```python
from build123d import *

# Parameters (mm, degrees)
F0_R     = 4
F1_DEPTH = 25


with BuildPart() as f1:
    # F0 (on Front) → F1 (new body)
    with BuildSketch(Plane.XZ):
        with BuildLine():
            ThreePointArc((1.7153142053, -12.3817485509), (9.425800432, -8.2100113408), (12.5, 0))
            ThreePointArc((12.5, 0), (0, 12.5), (-12.5, 0))
            ThreePointArc((-12.5, 0), (-8.8388347648, -8.8388347648), (0, -12.5))
            Line((0, -12.5), (1.7153142053, -12.3817485509))
        make_face()
        Circle(F0_R, mode=Mode.SUBTRACT)
        with BuildLine():
            ThreePointArc((-12.5, 0), (0, 12.5), (12.5, 0))
            ThreePointArc((12.5, 0), (9.425800432, -8.2100113408), (1.7153142053, -12.3817485509))
            Line((1.7153142053, -12.3817485509), (65.5502033349, -7.9810573416))
            ThreePointArc((65.5502033349, -7.9810573416), (57.0047370671, -0.2752646609), (65, 8))
            Line((65, 8), (21.9245263595, 11.0022438251))
            ThreePointArc((21.9245263595, 11.0022438251), (16.3684000055, 13.8215743024), (14.5197193706, 19.771493992))
            Line((14.5197193706, 19.771493992), (18.6307429943, 61.272344506))
            ThreePointArc((18.6307429943, 61.272344506), (0.0177077601, 46.0000082517), (-18.6237623762, 61.2376237624))
            Line((-18.6237623762, 61.2376237624), (-12.5, 0))
        make_face()
        with BuildLine():
            ThreePointArc((0, -12.5), (0.8596927108, -12.4704020963), (1.7153142053, -12.3817485509))
            Line((1.7153142053, -12.3817485509), (0, -12.5))
        make_face()
        with BuildLine():
            Line((-19, 65), (-18.6237623762, 61.2376237624))
            ThreePointArc((-18.6237623762, 61.2376237624), (0.0177077601, 46.0000082517), (18.6307429943, 61.272344506))
            Line((18.6307429943, 61.272344506), (19, 65))
            Line((19, 65), (18.4899446576, 69.3728648001))
            ThreePointArc((18.4899446576, 69.3728648001), (0, 84), (-18.4899446576, 69.3728648001))
            Line((-18.4899446576, 69.3728648001), (-19, 65))
        make_face()
        with Locations((0, 65)):
            Circle(F0_R, mode=Mode.SUBTRACT)
        with BuildLine():
            ThreePointArc((-19, 65), (-18.905706614, 63.1094293386), (-18.6237623762, 61.2376237624))
            Line((-18.6237623762, 61.2376237624), (-19, 65))
        make_face()
        with BuildLine():
            ThreePointArc((65, 8), (57.0047370671, -0.2752646609), (65.5502033349, -7.9810573416))
            ThreePointArc((65.5502033349, -7.9810573416), (70.8481461455, -5.4588631289), (73, 0))
            ThreePointArc((73, 0), (70.6568542495, 5.6568542495), (65, 8))
        make_face()
        with Locations((65, 0)):
            Circle(F0_R, mode=Mode.SUBTRACT)
        with BuildLine():
            ThreePointArc((-18.4899446576, 69.3728648001), (-18.8720553795, 67.2012554947), (-19, 65))
            Line((-19, 65), (-18.4899446576, 69.3728648001))
        make_face()
        with BuildLine():
            Line((19, 65), (18.6307429943, 61.272344506))
            ThreePointArc((18.6307429943, 61.272344506), (18.9074603912, 63.1270500395), (19, 65))
        make_face()
        with BuildLine():
            Line((-12.4158259076, 121.4481944044), (-18.4899446576, 69.3728648001))
            ThreePointArc((-18.4899446576, 69.3728648001), (0, 84), (18.4899446576, 69.3728648001))
            Line((18.4899446576, 69.3728648001), (12.4158259076, 121.4481944044))
            ThreePointArc((12.4158259076, 121.4481944044), (12.4789387338, 120.7253192936), (12.5, 120))
            ThreePointArc((12.5, 120), (-0.7253192936, 107.5210612662), (-12.4158259076, 121.4481944044))
        make_face()
        with Locations((-5, 100)):
            Circle(F0_R, mode=Mode.SUBTRACT)
        with BuildLine():
            Line((18.4899446576, 69.3728648001), (19, 65))
            ThreePointArc((19, 65), (18.8720553795, 67.2012554947), (18.4899446576, 69.3728648001))
        make_face()
        with BuildLine():
            ThreePointArc((12.4158259076, 121.4481944044), (0, 132.5), (-12.4158259076, 121.4481944044))
            ThreePointArc((-12.4158259076, 121.4481944044), (-0.7253192936, 107.5210612662), (12.5, 120))
            ThreePointArc((12.5, 120), (12.4789387338, 120.7253192936), (12.4158259076, 121.4481944044))
        make_face()
        with Locations((0, 120)):
            Circle(F0_R, mode=Mode.SUBTRACT)
    extrude(amount=F1_DEPTH)


solid = f1.part
```
For this review, take the finished solid that the model builds, in its own axes (mm). A direction names the side the tool comes from. Give positions to 0.01 mm unless a question says otherwise; leave off trailing zeros. Write each loop counter-clockwise with the first axis right and the second up, starting at its lowest first coordinate (ties: lowest second). Pieces come first, ordered by that corner, then holes. Notation, with made-up numbers: M 14,70.25 L 56,70.25 A25 ccw 56,96.25 Z; hole C -1,69.5 d11. An arc over 180 degrees is marked long. Answer as a JSON object with one key per item and string values. Group by question number.
Item 1: Draft analysis for pull direction X (two halves, no side actions). For faces 3 (the flat face through (33.19, -12.32, -10.21)), 4 (the cylindrical face through (-0.867, -12.325, 61.095)), 5 (the flat face through (6, 0, 45)), 6 (the cylindrical face through (68.695, -12.325, -1.532)), state which applies: +X half, -X half, draft (parallel to the pull), parting line (faces both ways), or undercut.
Item 2: Consider section A-A on y = -11. Write out the cut boundary in (x, z).
Item 3: For pin 1 Ø13 at (x, z) = (-5, 100) entering from -Y; pin 2 Ø7 at (x, z) = (0, 0) entering from +Y; pin 3 Ø2 at (x, y) = (8.5, -6) entering from -Z; pin 4 Ø10 at (x, y) = (58, -17.5) entering from -Z, all flat-tipped, find the tip position at first contact; note any pin that passes through.
Item 4: Consider section C-C on z = 120. Write out the cut boundary in (x, y).
Item 5: Consider section B-B on z = 100. Write out the cut boundary in (x, y), plus the area to 3 significant figures.
Item 6: Tool access review of faces 1 (the flat face through (16.546, -12.325, 40.231)), 2 (the cylindrical face through (-3.154, -12.325, 96.451)): name each direction out of +Z, -Z, +X, -X, +Y, -Y from which nothing blocks a thin tool from reaching the whole face with its end or side.
Item 7: Consider section D-D on x = 49.5. Write out the cut boundary in (y, z).
Item 8: For probe 1 along Z at (x, y) = (-3.5, -7); probe 2 along Z at (x, y) = (-5, -17.5); probe 3 along Z at (x, y) = (65, -11.75), list the stretches that pass through material, from the lowest coordinate up. Write a range as [from, to].
Check result:
{
 "1": {"face 3": "+X half", "face 4": "undercut", "face 5": "draft", "face 6": "undercut"},
 "2": {"outline": "M -18.62,61.24 L -12.5,0 A12.5 ccw 1.72,-12.38 L 65.55,-7.98 A8 ccw 65,8 L 21.92,11 A8 cw 14.52,19.77 L 18.63,61.27 A19 ccw 18.49,69.37 L 12.42,121.45 A12.5 ccw -12.42,121.45 L -18.49,69.37 A19 ccw Z; hole C -5,100 d8; hole C 0,0 d8; hole C 0,65 d8; hole C 0,120 d8; hole C 65,0 d8"},
 "3": {"pin 1": "stops at y = -25", "pin 2": "passes through", "pin 3": "stops at z = -11.98", "pin 4": "stops at z = -8.85"},
 "4": {"outline": "M -12.58,-25 L -4,-25 L -4,0 L -12.58,0 Z; M 4,-25 L 12.58,-25 L 12.58,0 L 4,0 Z"},
 "5": {"outline": "M -14.92,-25 L -9,-25 L -9,0 L -14.92,0 Z; M -1,-25 L 14.92,-25 L 14.92,0 L -1,0 Z", "area": "546 mm^2"},
 "6": {"face 1": "+X, +Y, -Y", "face 2": "+Y, -Y"},
 "7": {"outline": "M -25,-9.09 L 0,-9.09 L 0,9.08 L -25,9.08 Z"},
 "8": {"probe 1": "z = [-12, -1.94], [1.94, 63.06], [66.94, 96.29], [103.71, 118.06], [121.94, 132]", "probe 2": "z = [-11.46, 96], [104, 131.46]", "probe 3": "z = [-8.02, -4], [4, 8]"}
}
